```python
from build123d import *

# Parameters (mm, degrees)
SKETCH1_W           = 152.4
SKETCH1_H           = 38.1
BOSS_EXTRUDE1_DEPTH = 45.72
CUT_EXTRUDE1_REACH  = 162.247
SHELL1_T            = -2.032
CUT_EXTRUDE2_REACH  = 94.207
SKETCH4_W           = 33.02
SKETCH4_H           = 16.51
FILLET1_R           = 0.762
CHAMFER1_SIZE       = 5.08
CHAMFER1_SIZE_2     = 3.052371945


with BuildPart() as part:
    # Sketch1 → Boss-Extrude1 (new body)
    with BuildSketch(Plane(origin=(0, 0, 0), x_dir=(1, 0, 0), z_dir=(0, 1, 0))):
        Rectangle(SKETCH1_W, SKETCH1_H)
    extrude(amount=BOSS_EXTRUDE1_DEPTH)

    # Sketch3 → Cut-Extrude1 (cut, up to next)
    with BuildSketch(Plane(origin=(76.2, 0, 0), x_dir=(0, 0, -1), z_dir=(1, 0, 0)), mode=Mode.PRIVATE) as cut_extrude1_sk1:
        Polygon((-19.05, 15.63096767), (-0.970685408, 45.72), (-19.05, 45.72), align=None)
    cut_extrude1_tool1 = extrude(cut_extrude1_sk1.sketch, amount=-CUT_EXTRUDE1_REACH, mode=Mode.PRIVATE) & part.part
    add(cut_extrude1_tool1.solids().sort_by_distance((76.2, 35.690323, 13.023562))[0], mode=Mode.SUBTRACT)

    # Shell1
    shell1_openings = [part.faces().sort_by_distance(p)[0] for p in [
        (0, 0, 0),
    ]]
    offset(amount=SHELL1_T, openings=shell1_openings, kind=Kind.INTERSECTION)

    # Sketch4 → Cut-Extrude2 (cut, up to next)
    with BuildSketch(Plane(origin=(0, 12.556412247, 20.897379275), x_dir=(1, 0, 0), z_dir=(0, 0.5150380749100518, 0.8571673007021139)), mode=Mode.PRIVATE) as cut_extrude2_sk1:
        with Locations((-30.48, 20.249314041)):
            Rectangle(SKETCH4_W, SKETCH4_H)
    cut_extrude2_tool1 = extrude(cut_extrude2_sk1.sketch, amount=-CUT_EXTRUDE2_REACH, mode=Mode.PRIVATE) & part.part
    # Sketch4 → Cut-Extrude2 (cut, up to next)
    with BuildSketch(Plane(origin=(0, 12.556412247, 20.897379275), x_dir=(1, 0, 0), z_dir=(0, 0.5150380749100518, 0.8571673007021139)), mode=Mode.PRIVATE) as cut_extrude2_sk2:
        with Locations((30.48, 20.249314041)):
            Rectangle(SKETCH4_W, SKETCH4_H)
    cut_extrude2_tool2 = extrude(cut_extrude2_sk2.sketch, amount=-CUT_EXTRUDE2_REACH, mode=Mode.PRIVATE) & part.part
    add(cut_extrude2_tool1.solids().sort_by_distance((-30.48, 29.913462, 10.468212))[0], mode=Mode.SUBTRACT)
    add(cut_extrude2_tool2.solids().sort_by_distance((30.48, 29.913462, 10.468212))[0], mode=Mode.SUBTRACT)

    # Fillet1
    fillet1_edges = [part.edges().sort_by_distance(p)[0] for p in [
        (-76.2, 45.72, -9.039657296),
        (76.2, 45.72, -9.039657296),
        (76.2, 7.815483835, 19.05),
        (-76.2, 7.815483835, 19.05),
        (-76.2, 30.675483835, 10.010342704),
        (0, 45.72, 0.970685408),
        (76.2, 30.675483835, 10.010342704),
        (0, 15.63096767, 19.05),
        (-76.2, 22.86, -19.05),
        (76.2, 22.86, -19.05),
        (0, 45.72, -19.05),
    ]]
    fillet(fillet1_edges, radius=FILLET1_R)

    # Chamfer1
    # the kernel refuses this chamfer: 5.08, 3.052371945 mm, written as the material it takes off along each edge
    with BuildSketch(Plane(origin=(46.99, 21.790988669, 12.978086906), x_dir=(0, -0.8672541037770177, 0.4978657645208413), z_dir=(-1, 0, 0)), Plane(origin=(-13.97, 21.790988669, 12.978086906), x_dir=(0, -0.8672541037770181, 0.49786576452084075), z_dir=(-1, 0, 0))) as chamfer1_piece_1:
        Polygon((CHAMFER1_SIZE * 0.99980168408, CHAMFER1_SIZE * 0.0199146305808), (-CHAMFER1_SIZE_2 * 0.0199146305786, CHAMFER1_SIZE_2 * 0.999801683968), (0, 0), align=None)
    extrude(amount=33.02, mode=Mode.SUBTRACT)


solid = part.part
```
Source: CAD feature listing. Evaluate the final solid. Frame: model axes, mm. A direction names the side the tool comes from. Round coordinates to 2 decimals unless told otherwise and drop trailing zeros. Write each loop counter-clockwise with the first axis right and the second up, starting at its lowest first coordinate (ties: lowest second). Pieces come first, ordered by that corner, then holes. Notation, with made-up numbers: M -35,48.25 L 23,48.25 A13 ccw 23,66.25 Z; hole C -29.5,45.5 d7. An arc over 180 degrees is marked long. Answer as a JSON object with one key per item and string values. Group by question number.
(1) Mould query, pull axis X, two halves, no side actions, for faces 4 (the flat face through (0, 0, -18)), 5 (the flat face through (-1, 22, -17.018)), 6 (the flat face through (76.2, 22, -4)). Classes: +X half, -X half, draft (parallel to the pull), parting line (faces both ways), or undercut.
(2) Section query B-B on y = 6. Output: boundary loops of the cut face in (x, z), then the cut area to 3 significant figures.
(3) Section query A-A on x = 42. Output: boundary loops of the cut face in (y, z), then the cut area to 3 significant figures.
(4) Section query D-D on x = -61.5. Output: boundary loops of the cut face in (y, z).
(5) Reachability of faces 1 (the flat face through (-1, 8, 19.05)), 2 (the flat face through (-1, 43.688, -9)), 3 (the flat face through (-30, 19, 15.594)) from +Z, -Z, +X, -X, +Y, -Y: full face, straight path, thin tool, end or side. Return the list, or none.
(6) First-contact query: pin 1 (5 mm diameter, centred on x = -32, z = -7, fed in from -Y); pin 2 (1.5 mm diameter, centred on x = -35, z = 6, fed in from +Y); pin 3 (3.5 mm diameter, centred on y = 29, z = 12, fed in from -X); pin 4 (6 mm diameter, centred on x = 20.5, z = -0.5, fed in from -Y). Flat tips, straight axial feed; report the tip coordinate or a pass-through.
(7) Section query C-C on z = -3. Output: boundary loops of the cut face in (x, y).
(8) Ray query, line 1 (X direction, y = 21, z = 14); line 2 (Z direction, x = 41, y = 7); line 3 (X direction, y = 32, z = -3.5). Return the intervals inside material, ascending. Write a range as [from, to].
Computed values:
{
 "1": {"face 4": "draft", "face 5": "undercut", "face 6": "+X half"},
 "2": {"outline": "M -76.2,-18.29 A0.76 ccw -75.44,-19.05 L 75.44,-19.05 A0.76 ccw 76.2,-18.29 L 76.2,18.29 A0.76 ccw 75.44,19.05 L -75.44,19.05 A0.76 ccw -76.2,18.29 Z; hole M -74.17,-17.02 L 74.17,-17.02 L 74.17,17.02 L -74.17,17.02 Z", "area": "757 mm^2"},
 "3": {"outline": "M 0,-19.05 L 44.96,-19.05 A0.76 ccw 45.72,-18.29 L 45.72,0.54 A0.76 ccw 45.35,1.19 L 36.99,6.22 L 35.94,4.47 L 43.69,-0.18 L 43.69,-17.02 L 0,-17.02 Z; M 0,17.02 L 15.07,17.02 L 17.44,15.59 L 21.38,15.59 L 15.81,18.94 A0.76 ccw 15.42,19.05 L 0,19.05 Z", "area": "188 mm^2"},
 "4": {"outline": "M 0,-19.05 L 44.96,-19.05 A0.76 ccw 45.72,-18.29 L 45.72,0.54 A0.76 ccw 45.35,1.19 L 15.81,18.94 A0.76 ccw 15.42,19.05 L 0,19.05 L 0,17.02 L 15.07,17.02 L 43.69,-0.18 L 43.69,-17.02 L 0,-17.02 Z"},
 "5": {"face 1": "+Z, +X, -X, +Y, -Y", "face 2": "-Y", "face 3": "+Y, -Y"},
 "6": {"pin 1": "y = 43.69", "pin 2": "y = 38.6", "pin 3": "x = -76.2", "pin 4": "y = 39.23"},
 "7": {"outline": "M -76.2,0 L -74.17,0 L -74.17,43.69 L 74.17,43.69 L 74.17,0 L 76.2,0 L 76.2,44.96 A0.76 ccw 75.44,45.72 L -75.44,45.72 A0.76 ccw -76.2,44.96 Z"},
 "8": {"line 1": "[-76.2, -46.99], [-13.97, 13.97], [46.99, 76.2]", "line 2": "[-19.05, -17.02], [17.02, 19.05]", "line 3": "[-76.2, -74.17], [74.17, 76.2]"}
}
